Autodesk Inventor part; units mm, degrees
ref_plane "YZ Plane" through (0, 0, 0) normal (1, 0, 0) x (0, 1, 0)
ref_plane "XZ Plane" through (0, 0, 0) normal (0, 1, 0) x (-1, 0, 0)
ref_plane "XY Plane" through (0, 0, 0) normal (0, 0, 1) x (1, 0, 0)
sketch "Sketch1" plane through (0, 0, 0) normal (0, 1, 0) x (-1, 0, 0)
  circle A0 centre (0.2, 0) radius 7.35
  circle A1 centre (0.2, 0) radius 12.5
  line L0 (0.2, 0) -> (0.2, -3.5)
  line L1 (0.2, 0) -> (0.2, 3.5)
  line L2 (0.2, 3.5) -> (-0.5, 3.5)
  line L3 (-0.5, 3.5) -> (0.9, 3.5)
  line L4 (0.2, 0) -> (-0.5, 0)
  line L5 (-0.5, 0) -> (0.9, 0)
  line L6 (0.2, -3.5) -> (-0.5, -3.5)
  line L7 (-0.5, -3.5) -> (0.9, -3.5)
  circle A2 centre (-0.5, -3.5) radius 0.45
  circle A3 centre (0.9, -3.5) radius 0.45
  circle A4 centre (-0.5, 0) radius 0.45
  circle A5 centre (0.9, 0) radius 0.45
  circle A6 centre (-0.5, 3.5) radius 0.45
  circle A7 centre (0.9, 3.5) radius 0.45
  line L8 (0.9, -3.95) -> (-0.5, -3.95)
  line L9 (-0.5, -3.05) -> (0.9, -3.05)
  line L10 (0.9, -0.45) -> (-0.5, -0.45)
  line L11 (-0.5, 0.45) -> (0.9, 0.45)
  line L12 (-0.5, 3.05) -> (0.9, 3.05)
  line L13 (-0.5, 3.95) -> (0.9, 3.95)
  line L14 (1.35, 3.5) -> (1.35, -3.5)
  dimension "d0" = 14.7
  dimension "d1" = 25
  dimension "d14" = 3.5
  dimension "d15" = 3.5
  dimension "d16" = 0.7
  dimension "d17" = 1.4
  dimension "d18" = 0.7
  dimension "d19" = 1.4
  dimension "d20" = 0.7
  dimension "d21" = 1.4
  dimension "d22" = 0.9
  dimension "d23" = 0.9
  dimension "d24" = 0.9
  dimension "d25" = 0.9
  dimension "d26" = 0.9
  dimension "d27" = 0.9
extrude "Extrusion1" add sketch "Sketch1" along normal blind 15 contours A0 | L10 A5 L14 A3 L9 L0 | L1 L12 A7 L14 A5 L11
extrude "Extrusion2" add sketch "Sketch1" against normal blind 10 contours A0 | A1 | L10 A5 L14 A3 L9 L0 | L1 L12 A7 L14 A5 L11
properties part number "Kabelstopfen_Hinten_next try"
Geometry: final body of the model. Coordinates: model frame, mm. A direction names the side the tool comes from. Give positions to 0.01 mm unless a question says otherwise; leave off trailing zeros. Order: outer loops, then holes, each group sorted by start corner. A loop starts at its lowest first (then second) coordinate and runs counter-clockwise, first axis right, second up. Notation, with made-up numbers: (-19.75, 57.25) -> (-10.75, 57.25) arc R29 ccw to (-10.75, 90.25) -> close; hole circle Ø10 at (11, 3.25). An arc over 180 degrees is marked (long way). Answer as a JSON object with one key per item and string values.
Q1. Material intervals for probe 1 along Z at (x, y) = (0, -0.75); probe 2 along Z at (x, y) = (-0.75, 12.5); probe 3 along Y at (x, z) = (8, -9.25), sorted ascending.
Entries:
{"probe 1": "z = -12.5 to -3.95, -3.05 to -0.45, 0.45 to 3.05, 3.95 to 12.5", "probe 2": "z = -7.33 to -3.95, -3.05 to -0.45, 0.45 to 3.05, 3.95 to 7.33", "probe 3": "y = -10 to 0"}
Q2. Section C-C (z = 3.5). Output: boundary loops of the cut face in (x, y), plus the area to 3 significant figures.
Entries:
{"outline": "(-12.2, -10) -> (-1.35, -10) -> (-1.35, 15) -> (-6.66, 15) -> (-6.66, 0) -> (-12.2, 0) -> close; (0.95, -10) -> (11.8, -10) -> (11.8, 0) -> (6.26, 0) -> (6.26, 15) -> (0.95, 15) -> close", "area": "376 mm^2"}
Q3. Draft query along Z for faces 4 (the cylindrical face through (1.393, 7.395, 7.175)), 5 (the flat face through (0, 15, -2)), 6 (the flat face through (0, 2, 3.05)), 7 (the flat face through (0, 2, -3.05)). Return one class per face: released by +Z, released by -Z, zero draft, split by the parting line, or undercut.
Entries:
{"face 4": "split by the parting line", "face 5": "zero draft", "face 6": "undercut", "face 7": "undercut"}
Q4. Section A-A (y = -7). Output: boundary loops of the cut face in (x, z), plus the area to 3 significant figures.
Entries:
{"outline": "circle Ø25 at (-0.2, 0); hole (-0.9, -3.95) -> (0.5, -3.95) arc R0.45 ccw to (0.5, -3.05) -> (-0.9, -3.05) arc R0.45 ccw to start; hole (-0.9, -0.45) -> (0.5, -0.45) arc R0.45 ccw to (0.5, 0.45) -> (-0.9, 0.45) arc R0.45 ccw to start; hole (-0.9, 3.05) -> (0.5, 3.05) arc R0.45 ccw to (0.5, 3.95) -> (-0.9, 3.95) arc R0.45 ccw to start", "area": "485 mm^2"}
Q5. First-contact query: pin 1 (10 mm diameter, centred on x = 5, y = 6.5, fed in from +Z); pin 2 (1.5 mm diameter, centred on x = 0, y = 4, fed in from -Z); pin 3 (6 mm diameter, centred on x = -4.5, y = -5, fed in from -Z); pin 4 (0.7 mm diameter, centred on x = -0.5, y = -1.5, fed in from -Z). Flat tips, straight axial feed; report the tip coordinate or a pass-through.
Entries:
{"pin 1": "stops at z = 7.35", "pin 2": "stops at z = -7.35", "pin 3": "stops at z = -12.43", "pin 4": "stops at z = -12.5"}
Q6. Access query for faces 1 (the cylindrical face through (0.95, 2.32, -3.51)), 2 (the flat face through (-6, 0, -5)), 3 (the flat face through (-3, -10, 0)). Directions: +Z, -Z, +X, -X, +Y, -Y. A direction counts if a zero-diameter tool reaches every point of the face in a straight line with its end or side. Return the directions, or none.
Entries:
{"face 1": "+Y, -Y", "face 2": "+Y", "face 3": "+Z, -Z, +X, -X, -Y"}
Q7. Section B-B (x = -0.2). Output: boundary loops of the cut face in (y, z), plus the area to 3 significant figures.
Entries:
{"outline": "(-10, -12.5) -> (0, -12.5) -> (0, -7.35) -> (15, -7.35) -> (15, -3.95) -> (-10, -3.95) -> close; (-10, -3.05) -> (15, -3.05) -> (15, -0.45) -> (-10, -0.45) -> close; (-10, 0.45) -> (15, 0.45) -> (15, 3.05) -> (-10, 3.05) -> close; (-10, 3.95) -> (15, 3.95) -> (15, 7.35) -> (0, 7.35) -> (0, 12.5) -> (-10, 12.5) -> close", "area": "403 mm^2"}
Q8. Section D-D (y = 6). Output: boundary loops of the cut face in (x, z).
Entries:
{"outline": "circle Ø14.7 at (-0.2, 0); hole (-0.9, -3.95) -> (0.5, -3.95) arc R0.45 ccw to (0.5, -3.05) -> (-0.9, -3.05) arc R0.45 ccw to start; hole (-0.9, -0.45) -> (0.5, -0.45) arc R0.45 ccw to (0.5, 0.45) -> (-0.9, 0.45) arc R0.45 ccw to start; hole (-0.9, 3.05) -> (0.5, 3.05) arc R0.45 ccw to (0.5, 3.95) -> (-0.9, 3.95) arc R0.45 ccw to start"}
